from build123d import *

# Parameters (mm, degrees)
BOSS_EXTRUDE1_DEPTH = 2.54


with BuildPart() as part:
    # Sketch1 → Boss-Extrude1 (new body)
    with BuildSketch(Plane.XY):
        with BuildLine():
            Line((-19.895895452, 5.257641235), (-22.301043484, 3.549986133))
            Line((-22.301043484, 3.549986133), (-21.620166741, 2.584921984))
            ThreePointArc((-21.620166741, 2.584921984), (-20.673812198, 2.799001601), (-19.852490319, 2.282428882))
            Line((-19.852490319, 2.282428882), (-18.476919787, 3.25908396))
            Line((-18.476919787, 3.25908396), (-19.895895452, 5.257641235))
        make_face()
        with BuildLine():
            Line((-17.057944121, 1.260526684), (-18.476919787, 3.25908396))
            Line((-18.476919787, 3.25908396), (-19.852490319, 2.282428882))
            ThreePointArc((-19.852490319, 2.282428882), (-19.678061583, 1.933053448), (-19.618026709, 1.547198045))
            ThreePointArc((-19.618026709, 1.547198045), (-19.76048118, 0.962782884), (-20.155886678, 0.509474105))
            Line((-20.155886678, 0.509474105), (-19.475009935, -0.455590043))
            Line((-19.475009935, -0.455590043), (-17.057944121, 1.260526684))
        make_face()
        with BuildLine():
            Line((-21.9235631, 0.811967207), (-30.756728475, -5.459580209))
            ThreePointArc((-30.756728475, -5.459580209), (-30.582299739, -5.808955643), (-30.522264866, -6.194811046))
            ThreePointArc((-30.522264866, -6.194811046), (-30.663849348, -6.77754462), (-31.057034029, -7.230347437))
            Line((-31.057034029, -7.230347437), (-30.3732892, -8.193368322))
            Line((-30.3732892, -8.193368322), (-19.475009935, -0.455590043))
            Line((-19.475009935, -0.455590043), (-20.155886678, 0.509474105))
            ThreePointArc((-20.155886678, 0.509474105), (-21.102241221, 0.295394489), (-21.9235631, 0.811967207))
        make_face()
        with BuildLine():
            Line((-22.301043484, 3.549986133), (-33.211240531, -4.196253771))
            Line((-33.211240531, -4.196253771), (-32.527495703, -5.159274656))
            ThreePointArc((-32.527495703, -5.159274656), (-31.579916773, -4.942689532), (-30.756728475, -5.459580209))
            Line((-30.756728475, -5.459580209), (-21.9235631, 0.811967207))
            ThreePointArc((-21.9235631, 0.811967207), (-22.139830266, 1.761412556), (-21.620166741, 2.584921984))
            Line((-21.620166741, 2.584921984), (-22.301043484, 3.549986133))
        make_face()
        with BuildLine():
            Line((-33.211240531, -4.196253771), (-36.374783749, -6.442369456))
            Line((-36.374783749, -6.442369456), (-34.955808084, -8.440926731))
            Line((-34.955808084, -8.440926731), (-32.827801256, -6.930041884))
            ThreePointArc((-32.827801256, -6.930041884), (-33.04438638, -5.982462953), (-32.527495703, -5.159274656))
            Line((-32.527495703, -5.159274656), (-33.211240531, -4.196253771))
        make_face()
        with BuildLine():
            Line((-32.827801256, -6.930041884), (-34.955808084, -8.440926731))
            Line((-34.955808084, -8.440926731), (-33.536832418, -10.439484007))
            Line((-33.536832418, -10.439484007), (-30.3732892, -8.193368322))
            Line((-30.3732892, -8.193368322), (-31.057034029, -7.230347437))
            ThreePointArc((-31.057034029, -7.230347437), (-32.004612959, -7.446932561), (-32.827801256, -6.930041884))
        make_face()
    extrude(amount=BOSS_EXTRUDE1_DEPTH)


solid = part.part
For this review, take the finished solid that the model builds, in its own axes (mm). Round coordinates to 2 decimals unless told otherwise and drop trailing zeros. Loops run counter-clockwise (first coordinate to the right, second up) from the corner with the lowest first, then second, coordinate; pieces in that order, holes last. Notation, with made-up numbers: (28, -8.5) - (62, -8.5) arc R15 ccw to (62, 1.5) - close; hole circle Ø1 at (26, 46.25). An arc over 180 degrees is marked (long way). One line per item, written item: value. Start each with the question number.
Item 1: Take a section at C-C (y = -3). Give the boundary of the cut face in (x, z), plus the area to 3 significant figures.
Item 2: Take a section at A-A (z = 0.45). Give the boundary of the cut face in (x, y) (1 decimal).
Item 3: Clearance check with flat-ended pins moving along their axes: pin 1 Ø1.5 at (x, z) = (-28.5, 1) entering from +Y; pin 2 Ø1.5 at (x, z) = (-29, 1) entering from -Y. State where each tip first meets the part, or that it passes through.
Item 4: Take a section at D-D (x = -34). Give the boundary of the cut face in (y, z).
Item 5: For L1, parallel to X at y = -6.25, z = 1.7; L2, parallel to Y at x = -20, z = 0.7; L3, parallel to X at y = 0.5, z = 2.1, list the stretches that pass through material, from the lowest coordinate up.
Item 6: Take a section at B-B (y = -5.75). Give the boundary of the cut face in (x, z).
Answer below:
1. outline: (-31.53, 0) - (-23.06, 0) - (-23.06, 2.54) - (-31.53, 2.54) - close
1. area: 21.5 mm2
2. outline: (-36.4, -6.4) - (-33.5, -10.4) - (-17.1, 1.3) - (-19.9, 5.3) - close; hole circle Ø2.5 at (-31.8, -6.2); hole circle Ø2.5 at (-20.9, 1.5)
3. pin 1: stops at y = -0.32
3. pin 2: stops at y = -7.75
4. outline: (-9.79, 0) - (-4.76, 0) - (-4.76, 2.54) - (-9.79, 2.54) - close
5. L1: x = -36.1 to -33.06, -30.52 to -27.64
5. L2: y = -0.83 to 0.64, 2.46 to 5.18
5. L3: x = -26.6 to -21.61, -20.17 to -18.13
6. outline: (-35.4, 0) - (-32.98, 0) - (-32.98, 2.54) - (-35.4, 2.54) - close; (-30.6, 0) - (-26.93, 0) - (-26.93, 2.54) - (-30.6, 2.54) - close
